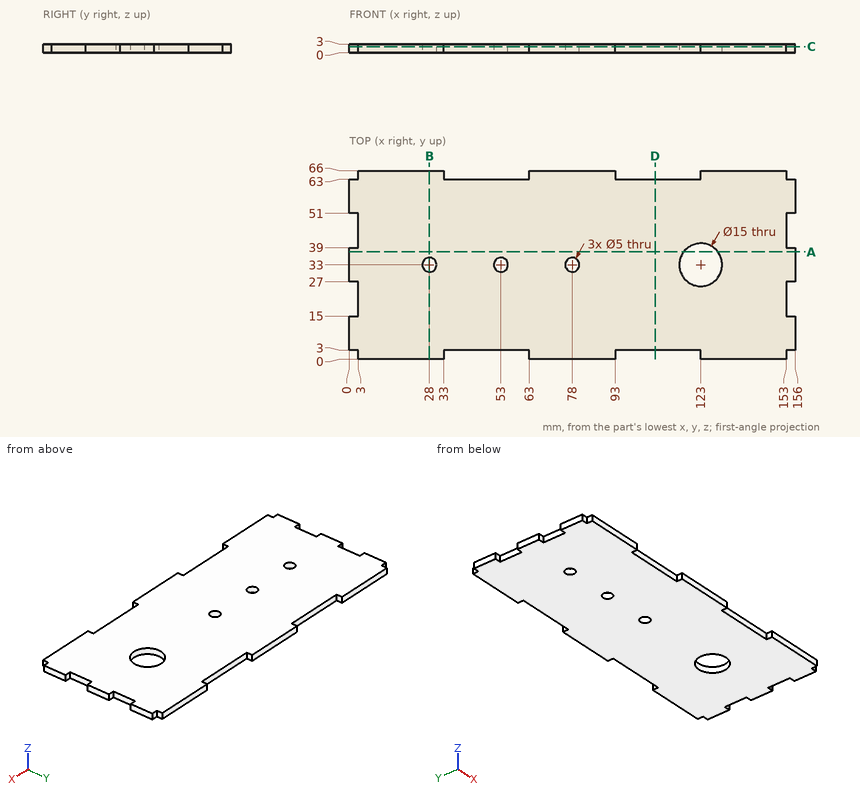
The drawing under review shows one solid part. Ordinate dimensions are in mm from its lowest x, y, z. Coordinates: 2 decimals unless noted, no trailing zeros. Order: outer loops, then holes, each group sorted by start corner. A loop starts at its lowest first (then second) coordinate and runs counter-clockwise, first axis right, second up. Notation, with made-up numbers: (-2.5, -1) -> (46.5, -1) arc R25 cw to (46.5, 25) -> close; hole circle Ø6 at (-30, 6.5). An arc over 180 degrees is marked (long way). Answer as CSV lines item,"result".
Q1. We need section A-A (y = 37.5). State the section outline as (x, z) points, plus the area to 3 significant figures.
Model answer:
outline,"(0, 0) -> (117, 0) -> (117, 3) -> (0, 3) -> close; (129, 0) -> (156, 0) -> (156, 3) -> (129, 3) -> close"
area,"432 mm2"
Q2. We need section B-B (x = 28). State the section outline as (y, z) points.
Model answer:
outline,"(0, 0) -> (30.5, 0) -> (30.5, 3) -> (0, 3) -> close; (35.5, 0) -> (66, 0) -> (66, 3) -> (35.5, 3) -> close"
Q3. Wall thickness on line 1 along Y through (x, z) = (28, 2.05); line 2 along Y through (x, z) = (53, 1.85); line 3 along X through (y, z) = (44.5, 1.35): over which ranges is each line inside the solid? List them lowest first. Write a range as [from, to].
Model answer:
line 1,"y = [0, 30.5], [35.5, 66]"
line 2,"y = [3, 30.5], [35.5, 63]"
line 3,"x = [3, 153]"
Q4. Clearance check with flat-ended pins moving along their axes: pin 1 Ø4.5 at (x, y) = (78, 33) entering from -Z; pin 2 Ø0.9 at (y, z) = (2, 2) entering from -X; pin 3 Ø1.5 at (x, z) = (155, 1) entering from +Y; pin 4 Ø0.9 at (y, z) = (64, 2) entering from +X. State where each tip first meets the part, or that it passes through.
Model answer:
pin 1,"passes through"
pin 2,"stops at x = 3"
pin 3,"stops at y = 63"
pin 4,"stops at x = 153"
Q5. We need section D-D (x = 107). State the section outline as (y, z) points.
Model answer:
outline,"(3, 0) -> (63, 0) -> (63, 3) -> (3, 3) -> close"
Q6. We need section C-C (z = 2.1). Count the separate pieces of the cut face and the enclosed holes in it, plus the area to 3 significant figures.
Model answer:
separate pieces,"1"
enclosed holes,"4"
area,"9,520 mm2"
